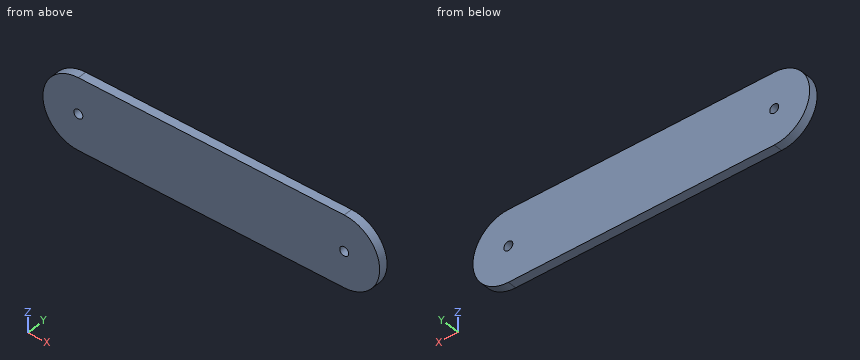
from build123d import *

# Parameters (mm, degrees)
BOSS_EXTRUDE1_DEPTH  = 3.175
M3_CLEARANCE_HOLE1_D = 3.2


with BuildPart() as part:
    # Sketch1 → Boss-Extrude1 (new body)
    with BuildSketch(Plane(origin=(0, 0, 0), x_dir=(1, 0, 0), z_dir=(0, 1, 0))):
        with BuildLine():
            Line((-47.625, 12.7), (47.625, 12.7))
            ThreePointArc((47.625, 12.7), (60.325, 0), (47.625, -12.7))
            Line((47.625, -12.7), (-47.625, -12.7))
            ThreePointArc((-47.625, -12.7), (-60.325, 0), (-47.625, 12.7))
        make_face()
    extrude(amount=BOSS_EXTRUDE1_DEPTH)

    # M3 Clearance Hole1 (through all)
    with Locations(Plane(origin=(0, 3.175, 0), x_dir=(1, 0, 0), z_dir=(0, 1, 0))):
        with Locations((-47.625, 0), (47.625, 0)):
            Hole(M3_CLEARANCE_HOLE1_D / 2)


solid = part.part
Geometry check sheet. Reference: the model listing, model coordinates, mm. Round coordinates to 2 decimals unless told otherwise and drop trailing zeros. Write each loop counter-clockwise with the first axis right and the second up, starting at its lowest first coordinate (ties: lowest second). Pieces come first, ordered by that corner, then holes. Notation, with made-up numbers: (44.25, 71.5) -> (93.25, 71.5) arc R10 ccw to (93.25, 86.5) -> close; hole circle Ø4 at (53.25, -26). An arc over 180 degrees is marked (long way). One line per item, written item: value. Start each with the question number.
(1) Cross-section at D-D, the plane z = -9.75. Record the cut outline in (x, y) (3 decimals).
(2) Scan lines: line 1 (X direction, y = 2.95, z = -0.5); line 2 (Z direction, x = 48.5, y = 2.9); line 3 (X direction, y = 0.65, z = -5.5). Record each from-to range of solid material in increasing order. Write a range as [from, to].
(3) Cross-section at B-B, the plane y = 2.3. Record the cut outline in (x, z) (3 decimals).
(4) Go/stop test with a flat-tipped pin: pin 1 Ø1.9 at (x, z) = (-47.625, 0) entering from +Y. Record where the tip stops, or that it passes through.
(5) Cross-section at A-A, the plane z = 0. Record the cut outline in (x, y) (3 decimals).
(6) Cross-section at C-C, the plane z = 10. Record the cut outline in (x, y) (3 decimals).
Answer:
1. outline: (-55.763, 0) -> (55.763, 0) -> (55.763, 3.175) -> (-55.763, 3.175) -> close
2. line 1: [-60.32, -49.14], [-46.11, 46.11], [49.14, 60.32]
2. line 2: [-12.67, -1.34], [1.34, 12.67]
2. line 3: [-59.07, 59.07]
3. outline: (-47.625, -12.7) -> (47.625, -12.7) arc R12.7 ccw to (47.625, 12.7) -> (-47.625, 12.7) arc R12.7 ccw to start; hole circle Ø3.2 at (-47.625, 0); hole circle Ø3.2 at (47.625, 0)
4. pin 1: through
5. outline: (-60.325, 0) -> (-49.225, 0) -> (-49.225, 3.175) -> (-60.325, 3.175) -> close; (-46.025, 0) -> (46.025, 0) -> (46.025, 3.175) -> (-46.025, 3.175) -> close; (49.225, 0) -> (60.325, 0) -> (60.325, 3.175) -> (49.225, 3.175) -> close
6. outline: (-55.454, 0) -> (55.454, 0) -> (55.454, 3.175) -> (-55.454, 3.175) -> close
